The listing builds one solid part. Answer for the finished solid, in the listing's coordinates (mm). Round coordinates to 2 decimals unless told otherwise and drop trailing zeros. Loops run counter-clockwise (first coordinate to the right, second up) from the corner with the lowest first, then second, coordinate; pieces in that order, holes last. Notation, with made-up numbers: (10, 43) - (21, 43) arc R27 cw to (21, 81) - close; hole circle Ø9 at (29, -31). An arc over 180 degrees is marked (long way). One line per question, with ' | ' between items. Start each with the question number.
from build123d import *

# Parameters (mm, degrees)
EXTRUDE1_DEPTH      = 24.37
EXTRUDE1_DEPTH_BACK = 24.37
SKETCH2_R           = 2.5
SKETCH3_R           = 2.5
EXTRUDE2_DEPTH      = 0.63
EXTRUDE2_TAPER      = 15
SKETCH4_R           = 2.5
EXTRUDE3_DEPTH      = 0.63
EXTRUDE3_TAPER      = 15


with BuildPart() as part:
    # Sketch2 → Extrude1 (new, two sides: drawn at the far end of the back side and taken through both)
    with BuildSketch(Plane(origin=(0, 0, 0), x_dir=(0, 0, -1), z_dir=(1, 0, 0)).offset(-EXTRUDE1_DEPTH_BACK)):
        Circle(SKETCH2_R)
    extrude(amount=EXTRUDE1_DEPTH + EXTRUDE1_DEPTH_BACK)

    # Sketch3 → Extrude2 (add)
    with BuildSketch(Plane(origin=(24.37, 0, 0), x_dir=(0, 0, -1), z_dir=(1, 0, 0))):
        Circle(SKETCH3_R)
    extrude(amount=EXTRUDE2_DEPTH, taper=EXTRUDE2_TAPER)

    # Sketch4 → Extrude3 (add)
    with BuildSketch(Plane.ZY.offset(24.37)):
        with Locations(Location((0, 0, 0), (0, 0, 180))):
            Circle(SKETCH4_R)
    extrude(amount=EXTRUDE3_DEPTH, taper=EXTRUDE3_TAPER)


solid = part.part
(1) Find section A-A on x = 12. Write down the section's boundary in (y, z).
(2) Consider L1, parallel to Y at x = 15, z = -0.2; L2, parallel to Z at x = 19.5, y = 0.95; L3, parallel to Z at x = -21.5, y = -1.55. Determine where each line is inside the solid, lowest interval first.
(3) Each of these flat-tipped pins is pushed along its axis until it touches: P1, Ø3, axis at x = 1, y = -1.5, coming from the -Z side; P2, Ø1, axis at x = -16.5, z = -2, coming from the -Y side. Where does it stop, or does it pass through?
Answer below:
1) outline: circle Ø5 at (0, 0)
2) L1: -2.49 to 2.49 | L2: -2.31 to 2.31 | L3: -1.96 to 1.96
3) P1: z = -2.5 | P2: y = -2
